from build123d import *

# Parameters (mm, degrees)
SKIZZE5_W                            = 2
SKIZZE5_H                            = 1.5
SCHNITT_LINEAR_AUSTRAGEN1_DEPTH      = 11
SCHNITT_LINEAR_AUSTRAGEN1_DEPTH_BACK = 11
F_6_0_6_DURCHMESSER_BOHRUNG1_D       = 6


with BuildPart() as part:
    # Skizze1 → Rotation1 (revolve)
    with BuildSketch(Plane(origin=(0, 0, 0), x_dir=(0, 0, -1), z_dir=(1, 0, 0)), mode=Mode.PRIVATE) as rotation1_sk:
        Polygon((10, 43), (10, 45), (0, 45), (0, -18), (5, -18), (5, 40), (10, 40), (10, 41), (9, 41), (9, 43), align=None)
    revolve(rotation1_sk.sketch.rotate(Axis((0, -18, 0), (0, -1, 0)), 180), axis=Axis((0, -18, 0), (0, -1, 0)))  # turned: the seam where the file's is

    # Skizze5 → Schnitt-Linear austragen1 (cut, two sides)
    with BuildSketch(Plane(origin=(0, 0, 0), x_dir=(0, 0, -1), z_dir=(1, 0, 0))) as schnitt_linear_austragen1_sk:
        with Locations((0, 44.25)):
            Rectangle(SKIZZE5_W, SKIZZE5_H)
    extrude(amount=SCHNITT_LINEAR_AUSTRAGEN1_DEPTH, mode=Mode.SUBTRACT)
    extrude(schnitt_linear_austragen1_sk.sketch, amount=-SCHNITT_LINEAR_AUSTRAGEN1_DEPTH_BACK, mode=Mode.SUBTRACT)

    # Ø6.0 (6) Durchmesser Bohrung1 (through all)
    with Locations(Plane(origin=(5, 0, 0), x_dir=(0, 0, 1), z_dir=(1, 0, 0))):
        with Locations((0, 0)):
            Hole(F_6_0_6_DURCHMESSER_BOHRUNG1_D / 2)


solid = part.part
Design review of the part built by this model. Coordinates are the model's own, in mm. A direction names the side the tool comes from. Round coordinates to 2 decimals unless told otherwise and drop trailing zeros. Write each loop counter-clockwise with the first axis right and the second up, starting at its lowest first coordinate (ties: lowest second). Pieces come first, ordered by that corner, then holes. Notation, with made-up numbers: M -30,-1 L -23,-1 A25 cw -23,27 Z; hole C 70,8 d1. An arc over 180 degrees is marked long. One line per item, written item: value. Start each with the question number.
1. Take a section at A-A on x = 0. State the section outline as (y, z) points.
2. Take a section at B-B on z = 0. State the section outline as (x, y) points, then the cut area to 3 significant figures.
3. Take a section at C-C on y = 0. State the section outline as (x, z) points, then the cut area to 3 significant figures.
4. Draft analysis for pull direction Z (two halves, no side actions). For faces 5 (the face through (0, 44, -10)), 6 (the face through (0, 45, 4)), 7 (the face through (0, 44, 1)), state which applies: pulls with the +Z half, pulls with the -Z half, needs draft (parallel to the pull), parting line crosses it, or undercut.
5. Take a section at D-D on z = -7.25. State the section outline as (x, y) points, then the cut area to 3 significant figures.
6. Clearance check with flat-ended pins moving along their axes: P1, Ø0.8, axis at x = -3.5, y = 44, coming from the +Z side; P2, Ø1, axis at x = -2.5, z = 0, coming from the +Y side; P3, Ø8, axis at x = 5, z = 4.5, coming from the -Y side; P4, Ø3.5, axis at y = 0, z = 0, coming from the +X side. State where each tip first meets the part, or that it passes through.
7. For faces 1 (the face through (-6.083, 42.014, -6.633)), 2 (the face through (-5, 40, -2)), 3 (the face through (-0.44, 40.51, -9.99)), 4 (the face through (0, 44, -1)), list the 3-axis set-ups (+Z, -Z, +X, -X, +Y, -Y) from which the entire face can be reached by the end or side of a thin tool; tool diameter is ignored.
8. To check wall thickness, follow probe 1 along Y at (x, z) = (-2.5, 0); probe 2 along Y at (x, z) = (-8, -5.5); probe 3 along Y at (x, z) = (4, 6). State the ranges of each line that lie inside material, in increasing order. Write a range as from..to.
Computed:
1. outline: M -18,-5 L 40,-5 L 40,-10 L 41,-10 L 41,-9 L 43,-9 L 43,-10 L 45,-10 L 45,-1 L 43.5,-1 L 43.5,1 L 45,1 L 45,10 L 43,10 L 43,9 L 41,9 L 41,10 L 40,10 L 40,5 L -18,5 Z; hole C 0,0 d6
2. outline: M -10,40 L -5,40 L -5,3 L 5,3 L 5,40 L 10,40 L 10,41 L 9,41 L 9,43 L 10,43 L 10,43.5 L -10,43.5 L -10,43 L -9,43 L -9,41 L -10,41 Z; M -5,-18 L 5,-18 L 5,-3 L -5,-3 Z
2. area: 586 mm²
3. outline: M -4,-3 A5 ccw 4,-3 Z; M -4,3 L 4,3 A5 ccw Z
3. area: 22.4 mm²
4. face 5: parting line crosses it
4. face 6: needs draft
4. face 7: undercut
5. outline: M -6.89,40 L 6.89,40 L 6.89,41 L 5.33,41 L 5.33,43 L 6.89,43 L 6.89,45 L -6.89,45 L -6.89,43 L -5.33,43 L -5.33,41 L -6.89,41 Z
5. area: 62.7 mm²
6. P1: stops at z = 9.51
6. P2: stops at y = 43.5
6. P3: stops at y = -18
6. P4: passes through
7. face 1: none
7. face 2: -Y
7. face 3: +Y, -Y
7. face 4: +X, -X, +Y
8. probe 1: y = -18..-3, 3..43.5
8. probe 2: y = 40..41, 43..45
8. probe 3: y = 40..45
